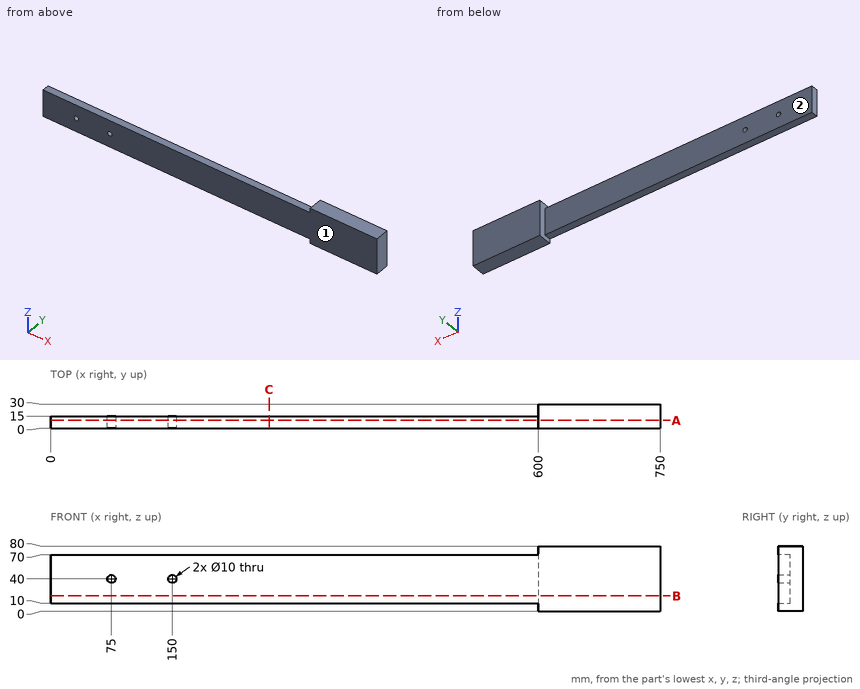
Can you work these out from the drawing? Everything is in mm from the part's minimum corner. A direction names the side the tool comes from. Give positions to 0.01 mm unless a question says otherwise; leave off trailing zeros. Write each loop counter-clockwise with the first axis right and the second up, starting at its lowest first coordinate (ties: lowest second). Pieces come first, ordered by that corner, then holes. Notation, with made-up numbers: (55, 35.5) -> (103, 35.5) arc R16 ccw to (103, 66.5) -> close; hole circle Ø2 at (-32.75, 62). An arc over 180 degrees is marked (long way). Write each question's results on one line, items separated by ' | '. Start each with the question number.
Q1. Suppose I cut it at C-C, the plane x = 269. List the corners of the cut face in (y, z) for me.
Q2. Suppose I cut it at B-B, the plane z = 19. List the corners of the cut face in (x, y) for me, and give its area (3 significant figures).
Q3. Suppose I cut it at A-A, the plane y = 10. List the corners of the cut face in (x, z) for me, and give its area (3 significant figures).
Q4. Which directions (+Z, -Z, +X, -X, +Y, -Y) give clear straight access to the entire face, cutting with the end or side of a thin tool? Please do the marked faces 1 and 2.
Q5. I need wall thicknesses on probe 1 along X at (y, z) = (9.75, 40); probe 2 along Z at (x, y) = (75, 8.5); probe 3 along Y at (x, z) = (397, 12). Which ranges of each line are inside material? Lowest first, please.
Q6. I'm going to push flat-ended pins straight in: pin 1 Ø12 at (x, y) = (185.5, 9.5) entering from +Z; pin 2 Ø13 at (x, z) = (150, 40) entering from -Y; pin 3 Ø13 at (x, z) = (75, 40) entering from +Y; pin 4 Ø12 at (y, z) = (25, 62.5) entering from -X. Where does each tip first touch, or does it pass through?
Outcome:
1) outline: (0, 10) -> (15, 10) -> (15, 70) -> (0, 70) -> close
2) outline: (0, 0) -> (750, 0) -> (750, 30) -> (600, 30) -> (600, 15) -> (0, 15) -> close | area: 13,500 mm2
3) outline: (0, 10) -> (600, 10) -> (600, 0) -> (750, 0) -> (750, 80) -> (600, 80) -> (600, 70) -> (0, 70) -> close; hole circle Ø10 at (75, 40); hole circle Ø10 at (150, 40) | area: 47,800 mm2
4) face 1: +Z, -Z, +X, -X, -Y | face 2: +Z, -Z, -X, +Y
5) probe 1: 0 to 70, 80 to 145, 155 to 750 | probe 2: 10 to 35, 45 to 70 | probe 3: 0 to 15
6) pin 1: z = 70 | pin 2: y = 0 | pin 3: y = 15 | pin 4: x = 600
